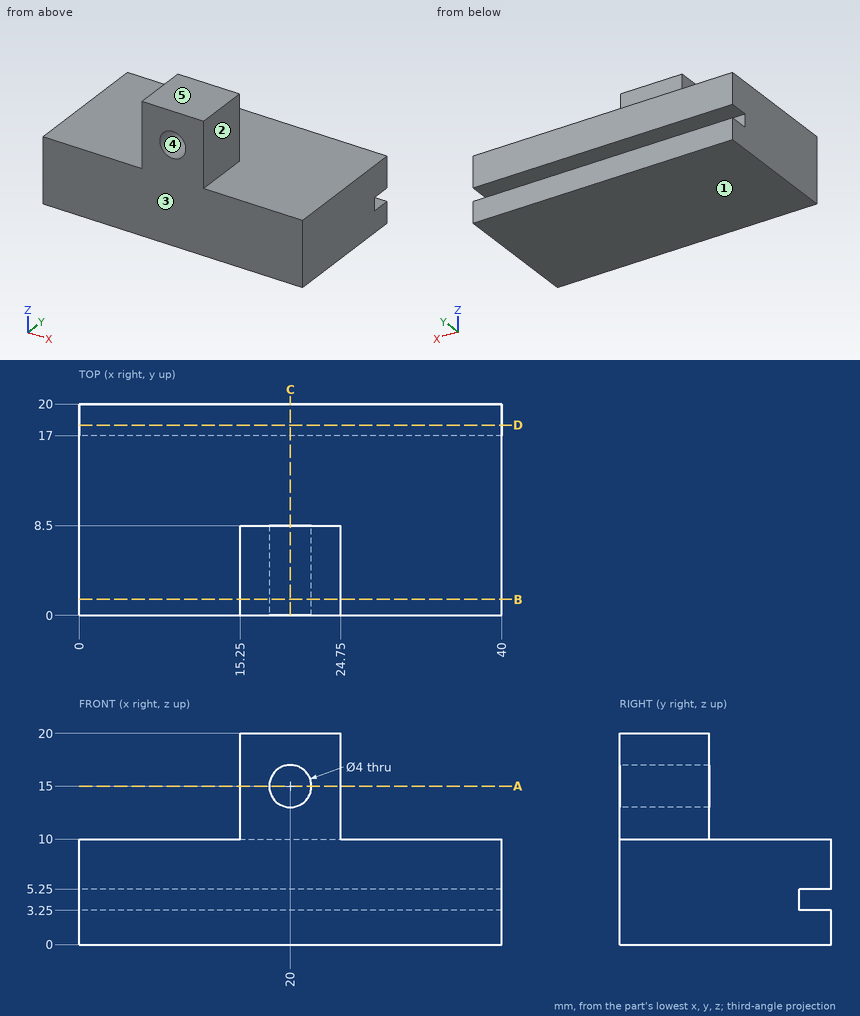
Part print with two shaded views. Sizes in mm from the minimum x, y, z corner. A direction names the side the tool comes from. Round coordinates to 2 decimals unless told otherwise and drop trailing zeros. Order: outer loops, then holes, each group sorted by start corner. A loop starts at its lowest first (then second) coordinate and runs counter-clockwise, first axis right, second up. Notation, with made-up numbers: M 76,-22.75 L 83,-22.75 A23 cw 83,16.25 Z; hole C 16,35 d7. An arc over 180 degrees is marked long. Use CSV: the item, a comma, the result in double quotes.
Item 1: Probe probe 1 along Z at (x, y) = (20, 4.75); probe 2 along Z at (x, y) = (36, 17.25); probe 3 along Y at (x, z) = (19.5, 10.5). List the from-to ranges inside material, lowest first.
Worked answers:
probe 1,"0 to 13, 17 to 20"
probe 2,"0 to 3.25, 5.25 to 10"
probe 3,"0 to 8.5"
Item 2: Which spindle directions (+Z, -Z, +X, -X, +Y, -Y) get a long thin tool onto all of the face, cutting with end or side? Do the marked faces 1 and 2. Say none if no direction does.
Worked answers:
face 1,"-Z, +X, -X, +Y, -Y"
face 2,"+Z, +X, +Y, -Y"
Item 3: Saw through at D-D (y = 18). List the corners of the cut face in (x, z), plus the area to 3 significant figures.
Worked answers:
outline,"M 0,0 L 40,0 L 40,3.25 L 0,3.25 Z; M 0,5.25 L 40,5.25 L 40,10 L 0,10 Z"
area,"320 mm²"
Item 4: Saw through at A-A (z = 15). List the corners of the cut face in (x, y), plus the area to 4 significant figures.
Worked answers:
outline,"M 15.25,0 L 18,0 L 18,8.5 L 15.25,8.5 Z; M 22,0 L 24.75,0 L 24.75,8.5 L 22,8.5 Z"
area,"46.75 mm²"
Item 5: Saw through at B-B (y = 1.5). List the corners of the cut face in (x, z), plus the area to 3 significant figures.
Worked answers:
outline,"M 0,0 L 40,0 L 40,10 L 24.75,10 L 24.75,20 L 15.25,20 L 15.25,10 L 0,10 Z; hole C 20,15 d4"
area,"482 mm²"
Item 6: Saw through at C-C (x = 20). List the corners of the cut face in (y, z), plus the area to 3 significant figures.
Worked answers:
outline,"M 0,0 L 20,0 L 20,3.25 L 17,3.25 L 17,5.25 L 20,5.25 L 20,10 L 8.5,10 L 8.5,13 L 0,13 Z; M 0,17 L 8.5,17 L 8.5,20 L 0,20 Z"
area,"245 mm²"
Item 7: Pull direction Z, two halves, no side cores. Call the marked faces 3, 4 and 5: released by +Z, released by -Z, zero draft, split by the parting line, or undercut.
Worked answers:
face 3,"zero draft"
face 4,"undercut"
face 5,"released by +Z"
Item 8: Pin check, flat tips, straight feed: pin 1 (0.9 mm diameter, centred on x = 25, y = 18, fed in from +Z); pin 2 (7.5 mm diameter, centred on x = 19.5, z = 15.5, fed in from +Y); pin 3 (1 mm diameter, centred on x = 21.5, z = 4.5, fed in from +Y). Stop position of each tip, or through.
Worked answers:
pin 1,"z = 10"
pin 2,"y = 8.5"
pin 3,"y = 17"
